Model file for the job. Use its own axes, mm. Face numbers are marked on the shaded views. A direction names the side the tool comes from. Round coordinates to 2 decimals unless told otherwise and drop trailing zeros. Order: outer loops, then holes, each group sorted by start corner. A loop starts at its lowest first (then second) coordinate and runs counter-clockwise, first axis right, second up. Notation, with made-up numbers: (2, -16.5) -> (38, -16.5) arc R21 cw to (38, 12.5) -> close; hole circle Ø5 at (74.5, -38.5). An arc over 180 degrees is marked (long way). Put each result on its own line as item: value. Start each with the question number.
Q1. Pull direction Y, two halves, no side cores. Call the marked faces 1, 2 and 3: released by +Y, released by -Y, zero draft, split by the parting line, or undercut.
Q2. Cut at C-C, the plane z = -1. List the corners of the cut face in (x, y).
Q3. 3-axis set-ups, long thin cutter, end or side, ignore diameter. For the marked faces 4, 5 and 6: which of +Z, -Z, +X, -X, +Y, -Y reach the whole face in a straight line?
Q4. Cut at D-D, the plane y = 35. List the corners of the cut face in (x, z), and give its area (3 significant figures).
Q5. Flat gauge pins, fed straight in: P1, Ø3, axis at x = 3.5, y = 37, coming from the +Z side; P2, Ø3, axis at x = -3, y = 37.5, coming from the -Z side; P3, Ø2, axis at y = 47.5, z = -2, coming from the -X side; P4, Ø7, axis at x = -0.5, z = -20, coming from the +Y side. Where does each tip first touch, or does it go through?
Q6. Probe L1, parallel to Y at x = -12, z = -8; L2, parallel to X at y = 2.25, z = 18; L3, parallel to X at y = 5.75, z = -18. List the from-to ranges inside material, lowest first.
Q7. Cut at A-A, the plane x = 16. List the corners of the cut face in (y, z).
Q8. Cut at B-B, the plane x = 7. List the corners of the cut face in (y, z), and give its area (3 significant figures).
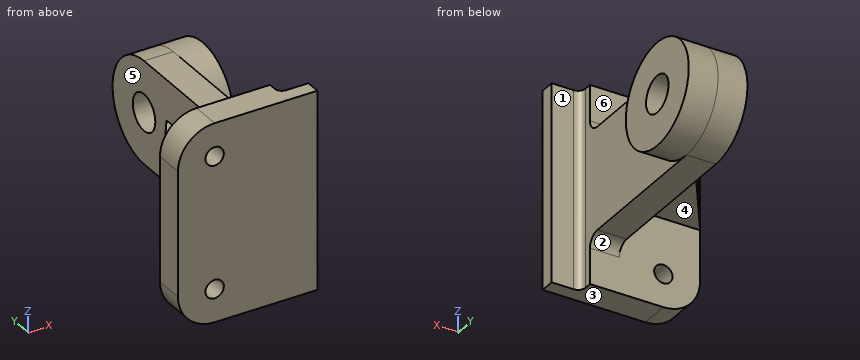
from build123d import *

# Parameters (mm, degrees)
Y_KSEKLIK_EKSTR_ZYON2_DEPTH      = 8
IZIM4_R                          = 2.5
KES_EKSTR_ZYON1_DEPTH            = 8
KES_EKSTR_ZYON2_DEPTH            = 54
IZIM13_W                         = 8
IZIM13_H                         = 41
Y_KSEKLIK_EKSTR_ZYON8_DEPTH      = 43
KES_EKSTR_ZYON7_DEPTH            = 43
IZIM15_R                         = 14
Y_KSEKLIK_EKSTR_ZYON9_DEPTH      = 8
Y_KSEKLIK_EKSTR_ZYON9_DEPTH_BACK = 8
IZIM16_R                         = 5
KES_EKSTR_ZYON8_DEPTH            = 16
FEDER12_REACH                    = 74.904
IZIM17_WALL_W                    = 187.469157084
IZIM17_WALL_H                    = 6


with BuildPart() as part:
    # Çizim3 → Yükseklik-Ekstrüzyon2 (new body)
    with BuildSketch(Plane(origin=(0, 0, 0), x_dir=(1, 0, 0), z_dir=(0, 1, 0))):
        with BuildLine():
            Line((-19, -17), (-19, 17))
            ThreePointArc((-19, 17), (-16.071067812, 24.071067812), (-9, 27))
            Line((-9, 27), (19, 27))
            Line((19, 27), (19, -27))
            Line((19, -27), (-9, -27))
            ThreePointArc((-9, -27), (-16.071067812, -24.071067812), (-19, -17))
        make_face()
    extrude(amount=Y_KSEKLIK_EKSTR_ZYON2_DEPTH)

    # Çizim4 → Kes-Ekstrüzyon1 (cut)
    with BuildSketch(Plane(origin=(0, 8, 0), x_dir=(1, 0, 0), z_dir=(0, 1, 0))):
        with Locations(Location((-9, -18, 0), (0, 0, 270))):
            Circle(IZIM4_R)
        with Locations(Location((-9, 18, 0), (0, 0, 90))):
            Circle(IZIM4_R)
    extrude(amount=-KES_EKSTR_ZYON1_DEPTH, mode=Mode.SUBTRACT)

    # Çizim5 → Kes-Ekstrüzyon2 (cut)
    with BuildSketch(Plane.XY.offset(27)):
        with BuildLine():
            Line((11, 8), (19, 8))
            Line((19, 8), (19, 4))
            Line((19, 4), (13, 4))
            ThreePointArc((13, 4), (11.585786438, 4.585786438), (11, 6))
            Line((11, 6), (11, 8))
        make_face()
    extrude(amount=-KES_EKSTR_ZYON2_DEPTH, mode=Mode.SUBTRACT)

    # Çizim13 → Yükseklik-Ekstrüzyon8 (add)
    with BuildSketch(Plane(origin=(0, 8, 0), x_dir=(1, 0, 0), z_dir=(0, 1, 0))):
        with Locations((7, 0)):
            Rectangle(IZIM13_W, IZIM13_H)
    extrude(amount=Y_KSEKLIK_EKSTR_ZYON8_DEPTH)

    # Çizim14 → Kes-Ekstrüzyon7 (cut)
    with BuildSketch(Plane.ZY.offset(-3)):
        with BuildLine():
            Line((20.5, 8), (20.5, 51))
            Line((20.5, 51), (14, 51))
            Line((14, 51), (14, 11.25))
            ThreePointArc((14, 11.25), (14.951902961, 8.951902961), (17.25, 8))
            Line((17.25, 8), (20.5, 8))
        make_face()
        with BuildLine():
            Line((-20.5, 51), (-14, 51))
            Line((-14, 51), (-14, 11.25))
            ThreePointArc((-14, 11.25), (-14.951902961, 8.951902961), (-17.25, 8))
            Line((-17.25, 8), (-20.5, 8))
            Line((-20.5, 8), (-20.5, 51))
        make_face()
    extrude(amount=-KES_EKSTR_ZYON7_DEPTH, mode=Mode.SUBTRACT)

    # Çizim15 → Yükseklik-Ekstrüzyon9 (add, two sides)
    with BuildSketch(Plane(origin=(11, 0, 0), x_dir=(0, 0, -1), z_dir=(1, 0, 0))) as y_kseklik_ekstr_zyon9_sk:
        with Locations((0, 51)):
            Circle(IZIM15_R)
    extrude(amount=Y_KSEKLIK_EKSTR_ZYON9_DEPTH)
    extrude(y_kseklik_ekstr_zyon9_sk.sketch, amount=-Y_KSEKLIK_EKSTR_ZYON9_DEPTH_BACK)

    # Çizim16 → Kes-Ekstrüzyon8 (cut)
    with BuildSketch(Plane(origin=(19, 0, 0), x_dir=(0, 0, -1), z_dir=(1, 0, 0))):
        with Locations((0, 51)):
            Circle(IZIM16_R)
    extrude(amount=-KES_EKSTR_ZYON8_DEPTH, mode=Mode.SUBTRACT)

    # Çizim17 wall → Feder12 (add, up to next)
    with BuildSketch(Plane(origin=(-8, 24.5, 0), x_dir=(0.554700196225, 0.832050294338, 0), z_dir=(-0.832050294338, 0.554700196225, 0)), mode=Mode.PRIVATE) as feder12_sk1:
        Rectangle(IZIM17_WALL_W, IZIM17_WALL_H)
    feder12_tool1 = extrude(feder12_sk1.sketch, amount=-FEDER12_REACH, mode=Mode.PRIVATE) - part.part
    add(feder12_tool1.solids().sort_by_distance((-8, 24.5, 0))[0])


solid = part.part
Ans:
1. face 1: undercut
1. face 2: released by +Y
1. face 3: zero draft
2. outline: (-19, 0) -> (19, 0) -> (19, 4) -> (13, 4) arc R2 cw to (11, 6) -> (11, 37.04) -> (19, 37.04) -> (19, 46.1) -> (3, 46.1) -> (3, 41) -> (-19, 8) -> close; (3, 55.9) -> (19, 55.9) -> (19, 64.96) -> (3, 64.96) -> close
3. face 4: -Z, -X, +Y
3. face 5: -X, +Y
3. face 6: +Z, -X, +Y
4. outline: (-1, -3) -> (3, -3) -> (3, -14) -> (11, -14) -> (11, 14) -> (3, 14) -> (3, 3) -> (-1, 3) -> close
4. area: 248 mm^2
5. P1: stops at z = 14
5. P2: passes through
5. P3: stops at x = 3
5. P4: stops at y = 8
6. L1: y = 0 to 8
6. L2: x = -18.95 to -11.5, -6.5 to 19
6. L3: x = -18.95 to -11.5, -6.5 to 11.02
7. outline: (0, -27) -> (4, -27) -> (4, 27) -> (0, 27) -> close; circle Ø28 at (51, 0); hole circle Ø10 at (51, 0)
8. outline: (0, -27) -> (8, -27) -> (8, -17.25) arc R3.25 cw to (11.25, -14) -> (51, -14) arc R14 ccw to (51, 14) -> (11.25, 14) arc R3.25 cw to (8, 17.25) -> (8, 27) -> (0, 27) -> close; hole circle Ø10 at (51, 0)
8. area: 1,870 mm^2
